Build history of the part. All positions in model axes, mm. Round coordinates to 2 decimals unless told otherwise and drop trailing zeros. Order: outer loops, then holes, each group sorted by start corner. A loop starts at its lowest first (then second) coordinate and runs counter-clockwise, first axis right, second up. Notation, with made-up numbers: (8, 27) - (63, 27) arc R20 cw to (63, 55) - close; hole circle Ø7 at (39.5, 21). An arc over 180 degrees is marked (long way). One line per question, with ' | ' between items. Start each with the question number.
from build123d import *

# Parameters (mm, degrees)
SKETCH042_R      = 4
EXTRUDE025_DEPTH = 30
SKETCH040_R      = 7
SKETCH044_W      = 60
SKETCH044_H      = 10.5
EXTRUDE027_DEPTH = 150
SKETCH046_R      = 3.5
SKETCH046_R_2    = 4
EXTRUDE029_DEPTH = 5


with BuildPart() as sweep011:
    # Sweep011: sweep along a path in Sketch
    with BuildLine(Plane.XY) as sweep011_path:
        ThreePointArc((0, 0), (65.583227, -3.22849), (127, 20))
    # Sketch042 → Sweep011 (sweep)
    with BuildSketch(Plane(origin=(0, 0, 0), x_dir=(0, -1, 0), z_dir=(-1, 0, 0))):
        Circle(SKETCH042_R)
    sweep(path=sweep011_path.line)


with BuildPart() as sweep011_1:
    # Sweep011 placement: moved
    add(sweep011.part.moved(Location((0, -3, 0))))


with BuildPart() as extrude025:
    # Sketch041 → Extrude025 (new body)
    with BuildSketch(Plane.XY.offset(-15)):
        Polygon((-8.268976, 21.973037), (10.121624, 21.973037), (-0.555824, -25), (-25.401805, -25), align=None)
        Polygon((105.81268, 45.885295), (155.276998, 45.885295), (207.473539, -4.114705), (135.506671, -4.114705), align=None)
    extrude(amount=EXTRUDE025_DEPTH)


with BuildPart() as motor_tube_outer003:
    # Sweep009: sweep along a path in Sketch
    with BuildLine(Plane.XY) as sweep009_path:
        ThreePointArc((0, 0), (65.583227, -3.22849), (127, 20))
    # Sketch040 → Sweep009 (sweep)
    with BuildSketch(Plane(origin=(0, 0, 0), x_dir=(0, -1, 0), z_dir=(-1, 0, 0))):
        Circle(SKETCH040_R)
    sweep(path=sweep009_path.line)

    # Cut010: cut Extrude025
    add(extrude025.part, mode=Mode.SUBTRACT)

    # Fusion010: union Sweep011
    add(sweep011_1.part)


with BuildPart() as cut013:
    # Sketch044 → Extrude027 (new body)
    with BuildSketch(Plane(origin=(-10, 0, 0), x_dir=(0, -1, 0), z_dir=(-1, 0, 0))):
        with Locations((-2, -5.25)):
            Rectangle(SKETCH044_W, SKETCH044_H)
    extrude(amount=-EXTRUDE027_DEPTH)

    # Cut013: cut Motor Tube Outer003
    add(motor_tube_outer003.part, mode=Mode.SUBTRACT)


with BuildPart() as motor_mold_bottom:
    # Sketch046 → Extrude029 (new body)
    with BuildSketch(Plane.XY):
        with Locations((19.376185, 19.084115)):
            Circle(SKETCH046_R)
        with Locations((114.867691, -14.293477)):
            Circle(SKETCH046_R_2)
    extrude(amount=EXTRUDE029_DEPTH)

    # Fusion013: union Cut013
    add(cut013.part)


solid = motor_mold_bottom.part
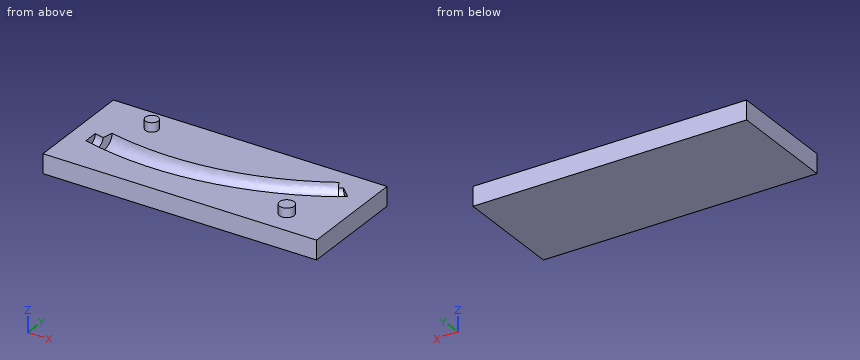
Item 1: Slice it at B-B (z = 2.75). Write the cut outline in (x, y), plus the area to 4 significant figures.
Item 2: Pin check, flat tip, straight feed: pin 1 (3 mm diameter, centred on x = 62.5, y = 11, fed in from +Z). Stop position of the tip, or through.
Item 3: Slice it at A-A (y = -21). Write the cut outline in (x, z).
Item 4: Wall check: line 1 along Z through (x, y) = (28, 21); line 2 along Y through (x, z) = (38.5, -6.25); line 3 along Y through (x, z) = (98, -0.5). Give the ranges that are in metal, low to high. Write a range as [from, to].
A:
1) outline: circle Ø7 at (19.38, 19.08); circle Ø8 at (114.87, -14.29) | area: 88.75 mm^2
2) pin 1: z = 0
3) outline: (-10, -10.5) - (140, -10.5) - (140, 0) - (-10, 0) - close
4) line 1: [-10.5, 0] | line 2: [-28, -8.23], [-2.13, 32] | line 3: [-28, -1.81], [12.66, 32]
